```python
from build123d import *

# Parameters (mm, degrees)
SALIENTE_EXTRUIR1_DEPTH = 11
SALIENTE_EXTRUIR2_DEPTH = 40
CROQUIS3_R              = 12
CROQUIS3_R_2            = 9
SALIENTE_EXTRUIR3_DEPTH = 3
CROQUIS3_2_R            = 9
CORTAR_EXTRUIR1_DEPTH   = 10
REDONDEO1_R             = 4


with BuildPart() as part:
    # Croquis1 → Saliente-Extruir1 (new body)
    with BuildSketch(Plane.XY):
        Polygon((-32.04318068, 26.167112062), (-30.431281855, 28.697286399), (-39.708587759, 34.607582091), (-41.320486584, 32.077407754), align=None)
    extrude(amount=-SALIENTE_EXTRUIR1_DEPTH)

    # Croquis2 → Saliente-Extruir2 (add)
    with BuildSketch(Plane.XY):
        Polygon((-26.214324626, 26.010788357), (-43.925544988, 37.294080133), (-45.537443813, 34.763905795), (-32.04318068, 26.167112062), (-27.826223451, 23.48061402), align=None)
    extrude(amount=SALIENTE_EXTRUIR2_DEPTH)

    # Croquis3 → Saliente-Extruir3 (add)
    with BuildSketch(Plane(origin=(4.219053857, 6.622587989, 0), x_dir=(0.843391446, -0.537299608, 0), z_dir=(0.537299608, 0.843391446, 0))):
        with Locations((-46.584523545, -26)):
            Circle(CROQUIS3_R)
        with Locations((-46.584523545, -26)):
            Circle(CROQUIS3_R_2, mode=Mode.SUBTRACT)
    extrude(amount=-SALIENTE_EXTRUIR3_DEPTH)

    # Croquis3<2> → Cortar-Extruir1 (cut)
    with BuildSketch(Plane(origin=(4.219053857, 6.622587989, 0), x_dir=(0.843391446, -0.537299608, 0), z_dir=(0.537299608, 0.843391446, 0))):
        with Locations((-46.584523545, -26)):
            Circle(CROQUIS3_2_R)
    extrude(amount=-CORTAR_EXTRUIR1_DEPTH, mode=Mode.SUBTRACT)

    # Redondeo1
    redondeo1_edges = [part.edges().sort_by_distance(p)[0] for p in [
        (-27.020274039, 24.745701189, 40),
        (-44.731494401, 36.028992964, 40),
    ]]
    fillet(redondeo1_edges, radius=REDONDEO1_R)


solid = part.part
```
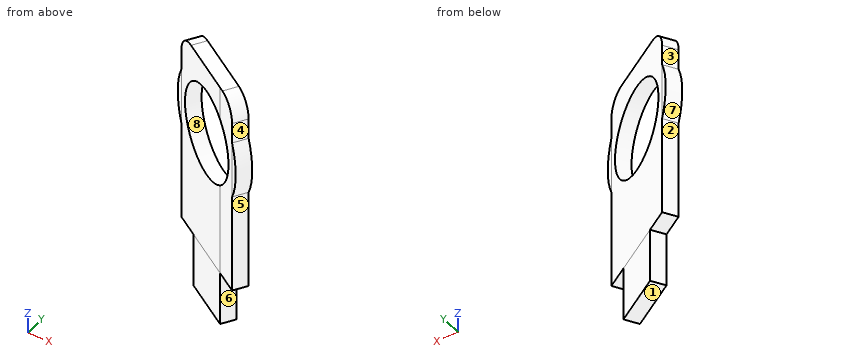
CAD build for the part. Positions are in the model's coordinates, mm. Face numbers are marked on the shaded views. A direction names the side the tool comes from. Round coordinates to 2 decimals unless told otherwise and drop trailing zeros. Write each loop counter-clockwise with the first axis right and the second up, starting at its lowest first coordinate (ties: lowest second). Pieces come first, ordered by that corner, then holes. Notation, with made-up numbers: (50, -40) -> (84, -40) arc R7 ccw to (84, -32) -> close; hole circle Ø7 at (75.5, 24). An arc over 180 degrees is marked (long way). Answer in a Markdown table with one row per item. Add a question column.
Item 1: Saw through at B-B, the plane z = 16. Write the cut outline in (x, y).
Item 2: Saw through at A-A, the plane z = 22. Write the cut outline in (x, y).
Item 3: Drop flat-ended pins along their axis: pin 1 Ø1.6 at (x, y) = (-42, 35.5) entering from -Z; pin 2 Ø1 at (x, z) = (-34, -4) entering from -Y; pin 3 Ø6 at (x, z) = (-35.5, 16) entering from -Y. Give the stop position or say it passes through.
Item 4: Drill centre lines: line 1 (Z direction, x = -30.25, y = 25.5); line 2 (Z direction, x = -33.5, y = 28.25); line 3 (Y direction, x = -38.75, z = 5.5). Where is each one in solid material? Low to high. Write a range as from..to.
Item 5: Mould opens along Z. For the marked faces 6, 7 and 8 say: pulls with the +Z half, pulls with the -Z half, needs draft (parallel to the pull), parting line crosses it, or undercut.
Item 6: Saw through at D-D, the plane z = -6. Write the cut outline in (x, y), then the cut area to 3 significant figures.
Item 7: Saw through at C-C, the plane z = 30.5. Write the cut outline in (x, y), then the cut area to 3 significant figures.
Item 8: Which spindle directions (+Z, -Z, +X, -X, +Y, -Y) get a long thin tool onto all of the face, cutting with end or side? Do the marked faces 1, 2, 3, 4 and 5. Say none if no direction does.
Findings below:
| question | item | result |
|---|---|---|
| 1 | outline | (-45.54, 34.76) -> (-27.83, 23.48) -> (-26.21, 26.01) -> (-43.93, 37.29) -> close |
| 2 | outline | (-46.22, 35.2) -> (-43.48, 33.45) -> (-41.87, 35.98) -> (-44.61, 37.73) -> close; (-29.88, 24.79) -> (-27.14, 23.04) -> (-25.53, 25.57) -> (-28.27, 27.32) -> close |
| 3 | pin 1 | stops at z = 0 |
| 3 | pin 2 | stops at y = 27.1 |
| 3 | pin 3 | stops at y = 26.46 |
| 4 | line 1 | z = 0..20.84, 31.16..39.9 |
| 4 | line 2 | z = -11..17.57, 34.43..40 |
| 4 | line 3 | y = 30.44..34 |
| 5 | face 6 | needs draft |
| 5 | face 7 | parting line crosses it |
| 5 | face 8 | undercut |
| 6 | outline | (-41.32, 32.08) -> (-32.04, 26.17) -> (-30.43, 28.7) -> (-39.71, 34.61) -> close |
| 6 | area | 33.0 mm^2 |
| 7 | outline | (-46.06, 35.1) -> (-43.26, 33.31) -> (-41.64, 35.84) -> (-44.45, 37.63) -> close; (-30.11, 24.93) -> (-27.3, 23.15) -> (-25.69, 25.68) -> (-28.5, 27.46) -> close |
| 7 | area | 20.0 mm^2 |
| 8 | face 1 | -Z, +X, -X, +Y, -Y |
| 8 | face 2 | -Z, -X, +Y |
| 8 | face 3 | +Z, -X, +Y |
| 8 | face 4 | +Z, +X, -Y |
| 8 | face 5 | -Z, +X, -Y |
